Autodesk Inventor part; units mm, degrees
ref_plane "YZ Plane" through (0, 0, 0) normal (1, 0, 0) x (0, 1, 0)
ref_plane "XZ Plane" through (0, 0, 0) normal (0, 1, 0) x (-1, 0, 0)
ref_plane "XY Plane" through (0, 0, 0) normal (0, 0, 1) x (1, 0, 0)
sketch "Sketch1" plane through (0, 0, 0) normal (0, 0, 1) x (1, 0, 0)
  circle A0 centre (0, 0) radius 23.495
  dimension "d0" = 46.99
extrude "Extrusion1" add sketch "Sketch1" along normal blind 3.175
sketch "Sketch2" plane through (0, 0, 0) normal (0, 0, -1) x (-1, 0, 0)
  line L0 (0, 0) -> (0, 8.3295)
  circle A0 centre (0, 8.3295) radius 1.5875
  circle A1 centre (-7.2136, -4.1648) radius 1.5875
  circle A2 centre (7.2136, -4.1648) radius 1.5875
  dimension "d3" = 3.175
  dimension "d6" = 360
  dimension "d8" = 14.4272
extrude "Extrusion2" cut sketch "Sketch2" against normal blind 3.175
sketch "Sketch3" plane through (0, 0, 3.175) normal (0, 0, 1) x (1, 0, 0)
  circle A0 centre (0, 0) radius 4.7625
  dimension "d11" = 9.525
extrude "Extrusion3" cut sketch "Sketch3" against normal blind 3.175
properties part number "pistonSpurGear" material "ABS Plastic"
Geometry: final body of the model. Coordinates: model frame, mm. Coordinates: 2 decimals unless noted, no trailing zeros. Order: outer loops, then holes, each group sorted by start corner. A loop starts at its lowest first (then second) coordinate and runs counter-clockwise, first axis right, second up. Notation, with made-up numbers: (0, -9) -> (7, -9) arc R14 ccw to (7, -4) -> close; hole circle Ø4 at (46.25, -10.75). An arc over 180 degrees is marked (long way). Use CSV: the item, a comma, the result in double quotes.
1) Pin query (flat end, axial travel): pin 1 Ø3.5 at (x, y) = (7.21, -4.16) entering from -Z. Return the tip coordinate at first contact, or that it passes through.
Findings:
pin 1,"stops at z = 0"
2) Section A-A on x = 0. Output: boundary loops of the cut face in (y, z) (1 decimal), then the cut area to 3 significant figures.
Findings:
outline,"(-23.5, 0) -> (-4.8, 0) -> (-4.8, 3.2) -> (-23.5, 3.2) -> close; (4.8, 0) -> (6.7, 0) -> (6.7, 3.2) -> (4.8, 3.2) -> close; (9.9, 0) -> (23.5, 0) -> (23.5, 3.2) -> (9.9, 3.2) -> close"
area,"109 mm^2"
3) Mould query, pull axis X, two halves, no side actions, for faces 1 (the cylindrical face through (8.8, -4.1, 1.6)), 2 (the flat face through (0, -5, 3.175)), 3 (the cylindrical face through (-5.093, 22.936, 1.565)). Classes: +X half, -X half, draft (parallel to the pull), parting line (faces both ways), or undercut.
Findings:
face 1,"undercut"
face 2,"draft"
face 3,"parting line"
4) Section B-B on y = 0. Output: boundary loops of the cut face in (x, z) (1 decimal).
Findings:
outline,"(-23.5, 0) -> (-4.8, 0) -> (-4.8, 3.2) -> (-23.5, 3.2) -> close; (4.8, 0) -> (23.5, 0) -> (23.5, 3.2) -> (4.8, 3.2) -> close"
5) Line query: line 1 (Y direction, x = 0, z = 1.4) (1 decimal); line 2 (X direction, y = 9, z = 2.9); line 3 (Y direction, x = -8, z = 0.4). Output: solid intervals per line, ascending.
Findings:
line 1,"y = -23.5 to -4.8, 4.8 to 6.7, 9.9 to 23.5"
line 2,"x = -21.7 to -1.44, 1.44 to 21.7"
line 3,"y = -22.09 to -5.54, -2.79 to 22.09"
6) Section D-D on y = -17.5. Output: boundary loops of the cut face in (x, z) (3 decimals), then the cut area to 3 significant figures.
Findings:
outline,"(-15.677, 0) -> (15.677, 0) -> (15.677, 3.175) -> (-15.677, 3.175) -> close"
area,"99.5 mm^2"
7) Section C-C on z = 2.15. Output: boundary loops of the cut face in (x, y) (1 decimal), then the cut area to 3 significant figures.
Findings:
outline,"circle Ø47 at (0, 0); hole circle Ø3.2 at (-7.2, -4.2); hole circle Ø9.5 at (0, 0); hole circle Ø3.2 at (0, 8.3); hole circle Ø3.2 at (7.2, -4.2)"
area,"1,640 mm^2"
